Source: three-view drawing plus pictorial views. Frame: mm from the lowest corner of the part. A direction names the side the tool comes from. Give positions to 0.01 mm unless a question says otherwise; leave off trailing zeros. Loops run counter-clockwise (first coordinate to the right, second up) from the corner with the lowest first, then second, coordinate; pieces in that order, holes last. Notation, with made-up numbers: M 19,42.25 L 54,42.25 A33 cw 54,79.25 Z; hole C 66,11 d10. An arc over 180 degrees is marked long. Write item = value, one per line.
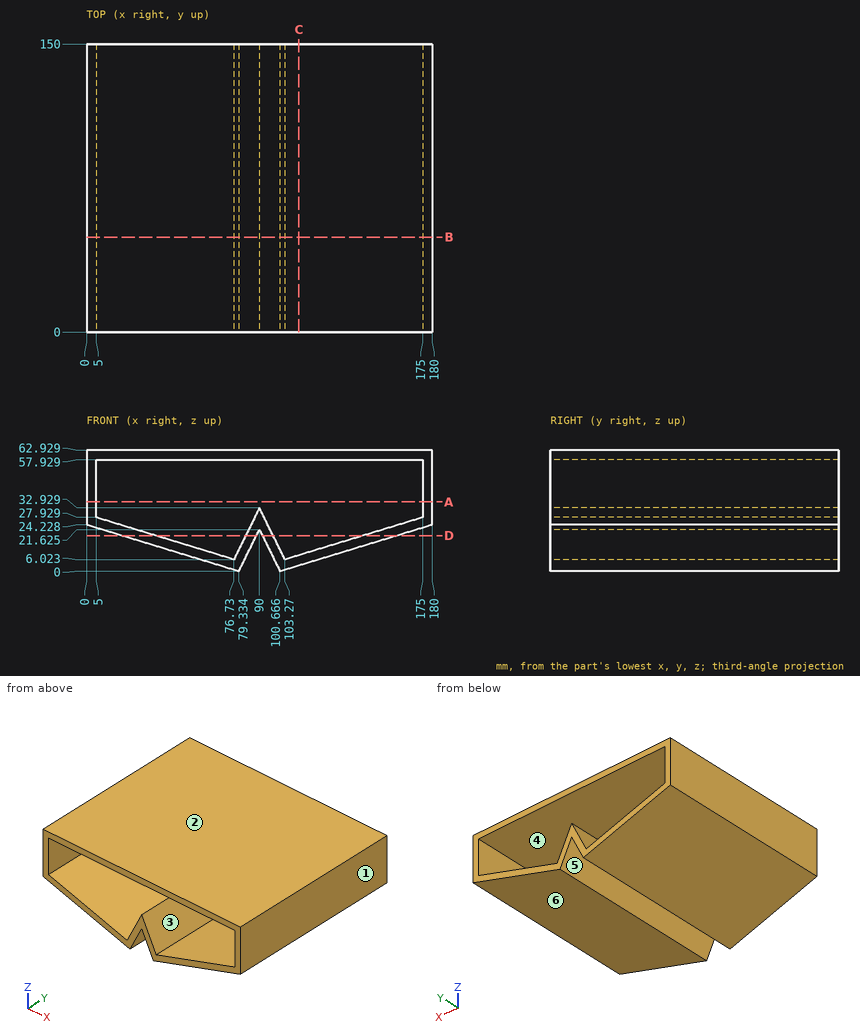
1. Cut plane B-B, the plane y = 49.5. Return the cut outline in (x, z) (1 decimal).
Derived:
outline = M 0,24.2 L 79.3,0 L 90,21.6 L 100.7,0 L 180,24.2 L 180,62.9 L 0,62.9 Z; hole M 5,27.9 L 76.7,6 L 90,32.9 L 103.3,6 L 175,27.9 L 175,57.9 L 5,57.9 Z
2. Cut plane C-C, the plane x = 110.5. Return the cut outline in (y, z), then the cut area to 3 significant figures.
Derived:
outline = M 0,3 L 150,3 L 150,8.23 L 0,8.23 Z; M 0,57.93 L 150,57.93 L 150,62.93 L 0,62.93 Z
area = 1,530 mm²
3. Reachability of the marked faces 4, 5 and 6 from +Z, -Z, +X, -X, +Y, -Y: full face, straight path, thin tool, end or side. Return the list, or none.
Derived:
face_4 = +Y, -Y
face_5 = -Z, +Y, -Y
face_6 = -Z, +X, +Y, -Y
4. Pull-direction query (Z, two-part tool) for the marked faces 1, 2 and 3; classes: +Z half, -Z half, draft (parallel to the pull), parting line (faces both ways), or undercut.
Derived:
face_1 = draft
face_2 = +Z half
face_3 = undercut
5. Cut plane D-D, the plane z = 18.5. Return the cut outline in (x, y) (1 decimal).
Derived:
outline = M 18.8,0 L 35.9,0 L 35.9,150 L 18.8,150 Z; M 82.9,0 L 88.5,0 L 88.5,150 L 82.9,150 Z; M 91.5,0 L 97.1,0 L 97.1,150 L 91.5,150 Z; M 144.1,0 L 161.2,0 L 161.2,150 L 144.1,150 Z
6. Material intervals for probe 1 along X at (y, z) = (33.5, 49); probe 2 along X at (y, z) = (128.5, 30.5); probe 3 along Z at (x, y) = (158, 46.5), sorted ascending. Write a range as from..to.
Derived:
probe_1 = 0..5, 175..180
probe_2 = 0..5, 88.8..91.2, 175..180
probe_3 = 17.51..22.74, 57.93..62.93
7. Cut plane A-A, the plane z = 36. Return the cut outline in (x, y), then the cut area to 3 significant figures.
Derived:
outline = M 0,0 L 5,0 L 5,150 L 0,150 Z; M 175,0 L 180,0 L 180,150 L 175,150 Z
area = 1,500 mm²
